Build history of the part. All positions in model axes, mm. A direction names the side the tool comes from. Round coordinates to 2 decimals unless told otherwise and drop trailing zeros. Loops run counter-clockwise (first coordinate to the right, second up) from the corner with the lowest first, then second, coordinate; pieces in that order, holes last. Notation, with made-up numbers: (-10.5, 80) - (25.5, 80) arc R15 cw to (25.5, 97) - close; hole circle Ø5 at (39, 57). An arc over 180 degrees is marked (long way). Use a Markdown table: item, result.
from build123d import *

# Parameters (mm, degrees)
SKETCH1_W                  = 66
SKETCH1_H                  = 60
BOSS_EXTRUDE1_DEPTH        = 20
CUT_EXTRUDE1_REACH         = 62
SKETCH2_W                  = 30
SKETCH2_H                  = 9.4
M6_TAPPED_HOLE1_AT_2_COUNT = 2
M6_TAPPED_HOLE1_AT_2_PITCH = 36
SKETCH7_R                  = 3.5
CUT_EXTRUDE2_DEPTH         = 21
SKETCH9_R                  = 6
CUT_EXTRUDE3_DEPTH         = 6


with BuildPart() as part:
    # Sketch1 → Boss-Extrude1 (new body)
    with BuildSketch(Plane.XY):
        Rectangle(SKETCH1_W, SKETCH1_H)
        with BuildLine():
            Line((10.5, -3), (6.873863542, -3))
            ThreePointArc((6.873863542, -3), (-7.5, 0), (6.873863542, 3))
            Line((6.873863542, 3), (10.5, 3))
            Line((10.5, 3), (10.5, -3))
        make_face(mode=Mode.SUBTRACT)
    extrude(amount=BOSS_EXTRUDE1_DEPTH)

    # Sketch2 → Cut-Extrude1 (cut, up to next)
    with BuildSketch(Plane(origin=(0, 30, 0), x_dir=(1, 0, 0), z_dir=(0, 1, 0)), mode=Mode.PRIVATE) as cut_extrude1_sk1:
        with Locations((0, -4.7)):
            Rectangle(SKETCH2_W, SKETCH2_H)
    cut_extrude1_tool1 = extrude(cut_extrude1_sk1.sketch, amount=-CUT_EXTRUDE1_REACH, mode=Mode.PRIVATE) & part.part
    add(cut_extrude1_tool1.solids().sort_by_distance((0, 30, 4.7))[0], mode=Mode.SUBTRACT)

    # Sketch5 → M6 Tapped Hole1 (revolve, cut)
    with BuildSketch(Plane(origin=(-33, 18, 10), x_dir=(0, 0, 1), z_dir=(0, 1, 0))):
        Polygon((0, 0), (0, 29.502151548), (2.5, 28), (2.5, 0), align=None)
    m6_tapped_hole1 = revolve(axis=Axis((-39.35, 18, 10), (1, 0, 0)), mode=Mode.SUBTRACT)

    # M6 Tapped Hole1 at 2: M6 Tapped Hole1 ×2
    with Locations(*[(0, -i * M6_TAPPED_HOLE1_AT_2_PITCH, 0) for i in range(1, M6_TAPPED_HOLE1_AT_2_COUNT)]):
        add(m6_tapped_hole1, mode=Mode.SUBTRACT)

    # Mirror1: M6 Tapped Hole1 across plane
    add(m6_tapped_hole1.mirror(Plane(origin=(0, 0, 0), x_dir=(0, 0, 1), z_dir=(1, 0, 0))), mode=Mode.SUBTRACT)

    # Mirror1 copy 1 sketch → Mirror1 copy 1 (revolve, cut)
    with BuildSketch(Plane(origin=(33, -18, 10), x_dir=(0, 0, 1), z_dir=(0, 1, 0))):
        Polygon((0, 0), (0, -29.502151548), (2.5, -28), (2.5, 0), align=None)
    revolve(axis=Axis((39.35, -18, 10), (1, 0, 0)), mode=Mode.SUBTRACT)

    # Sketch7 → Cut-Extrude2 (cut, through all)
    with BuildSketch(Plane.XY.offset(20)):
        with Locations((0, 23)):
            Circle(SKETCH7_R)
        with Locations((23, 0)):
            Circle(SKETCH7_R)
        with Locations((0, -23)):
            Circle(SKETCH7_R)
        with Locations((-23, 0)):
            Circle(SKETCH7_R)
    extrude(amount=-CUT_EXTRUDE2_DEPTH, mode=Mode.SUBTRACT)

    # Sketch9 → Cut-Extrude3 (cut)
    with BuildSketch(Plane(origin=(0, 0, 0), x_dir=(-1, 0, 0), z_dir=(0, 0, -1))):
        with Locations((23, 0)):
            Circle(SKETCH9_R)
        with Locations((-23, 0)):
            Circle(SKETCH9_R)
    extrude(amount=-CUT_EXTRUDE3_DEPTH, mode=Mode.SUBTRACT)


solid = part.part
Q1. Pull direction Z, two halves, no side cores. Call faces 5 (the face through (3.926, 17.786, 10.679)), 6 (the face through (19.2, 18.96, 12.31)), 7 (the face through (-30, 0, 0)), 8 (the face through (-18.24, -3.65, 2.96)): pulls with the +Z half, pulls with the -Z half, needs draft (parallel to the pull), parting line crosses it, or undercut.
Results found:
| item | result |
|---|---|
| face 5 | undercut |
| face 6 | undercut |
| face 7 | pulls with the -Z half |
| face 8 | needs draft |
Q2. Probe line 1 (Y direction, x = 18.5, z = 10); line 2 (Y direction, x = 0, z = 12.5); line 3 (Z direction, x = 25.5, y = -18). List the from-to ranges inside material, lowest first.
Results found:
| item | result |
|---|---|
| line 1 | y = -30 to -20.5, -15.5 to 15.5, 20.5 to 30 |
| line 2 | y = -30 to -26.5, -19.5 to -7.5, 7.5 to 19.5, 26.5 to 30 |
| line 3 | z = 0 to 7.5, 12.5 to 20 |
Q3. Drop flat-ended pins along their axis: pin 1 (15 mm diameter, centred on x = 1, y = 13, fed in from -Z); pin 2 (4.5 mm diameter, centred on y = -18, z = 10, fed in from +X); pin 3 (4 mm diameter, centred on y = 18, z = 10, fed in from -X). Give the stop position or say it passes through.
Results found:
| item | result |
|---|---|
| pin 1 | stops at z = 9.4 |
| pin 2 | stops at x = 4.85 |
| pin 3 | stops at x = -4.7 |
Q4. Cut at C-C, the plane z = 17.25. List the corners of the cut face in (x, y).
Results found:
| item | result |
|---|---|
| outline | (-33, -30) - (33, -30) - (33, 30) - (-33, 30) - close; hole circle Ø7 at (-23, 0); hole circle Ø7 at (0, -23); hole circle Ø7 at (0, 23); hole (6.87, -3) - (10.5, -3) - (10.5, 3) - (6.87, 3) arc R7.5 ccw (long way) to start; hole circle Ø7 at (23, 0) |
Q5. Cut at D-D, the plane y = 24. List the corners of the cut face in (x, z).
Results found:
| item | result |
|---|---|
| outline | (-33, 0) - (-15, 0) - (-15, 9.4) - (-3.35, 9.4) - (-3.35, 20) - (-33, 20) - close; (3.35, 9.4) - (15, 9.4) - (15, 0) - (33, 0) - (33, 20) - (3.35, 20) - close |
Q6. Cut at B-B, the plane y = 0. List the corners of the cut face in (x, z), plus the area to 3 significant figures.
Results found:
| item | result |
|---|---|
| outline | (-33, 0) - (-29, 0) - (-29, 6) - (-26.5, 6) - (-26.5, 20) - (-33, 20) - close; (-19.5, 6) - (-17, 6) - (-17, 0) - (-15, 0) - (-15, 9.4) - (-7.5, 9.4) - (-7.5, 20) - (-19.5, 20) - close; (10.5, 9.4) - (15, 9.4) - (15, 0) - (17, 0) - (17, 6) - (19.5, 6) - (19.5, 20) - (10.5, 20) - close; (26.5, 6) - (29, 6) - (29, 0) - (33, 0) - (33, 20) - (26.5, 20) - close |
| area | 507 mm2 |
Q7. Which spindle directions (+Z, -Z, +X, -X, +Y, -Y) get a long thin tool onto all of the face, cutting with end or side? Do faces 1 (the face through (15, 0, 5)), 2 (the face through (20, -3, 6)), 3 (the face through (-19.196, -18.751, 12.385)), 4 (the face through (9, -3, 15)). Say none if no direction does.
Results found:
| item | result |
|---|---|
| face 1 | -Z, +Y, -Y |
| face 2 | -Z |
| face 3 | -X |
| face 4 | +Z, -Z |
Q8. Cut at A-A, the plane x = -23. List the corners of the cut face in (y, z).
Results found:
| item | result |
|---|---|
| outline | (-30, 0) - (-6, 0) - (-6, 6) - (-3.5, 6) - (-3.5, 20) - (-30, 20) - close; (3.5, 6) - (6, 6) - (6, 0) - (30, 0) - (30, 20) - (3.5, 20) - close; hole circle Ø5 at (-18, 10); hole circle Ø5 at (18, 10) |
